Drawing for the job (mm, zero at the part's lowest x, y, z). A direction names the side the tool comes from. Round coordinates to 2 decimals unless told otherwise and drop trailing zeros. Loops run counter-clockwise (first coordinate to the right, second up) from the corner with the lowest first, then second, coordinate; pieces in that order, holes last. Notation, with made-up numbers: M 85.5,30.5 L 113.5,30.5 A8 ccw 113.5,37.5 Z; hole C 21.25,11.25 d3. An arc over 180 degrees is marked long. Use a Markdown table: item, result. Add a question column.
Q1. Cut at A-A (y = 31). Give the cut face in (x, z).
Q2. Tool access for the marked faces 1 and 2: list every direction of +Z, -Z, +X, -X, +Y, -Y with a clear straight run to the whole face (end or side of a thin tool).
Q3. Mould opens along X. For the marked faces 3, 4 and 5 say: +X half, -X half, draft (parallel to the pull), parting line (faces both ways), or undercut.
Q4. Cut at B-B (x = 61.5). Give the cut face in (y, z).
Q5. Probe line 1 (X direction, y = 73.5, z = 45); line 2 (Y direction, x = 60.5, z = 44); line 3 (Z direction, x = 43, y = 35). List the from-to ranges inside material, lowest first. Write a range as from..to.
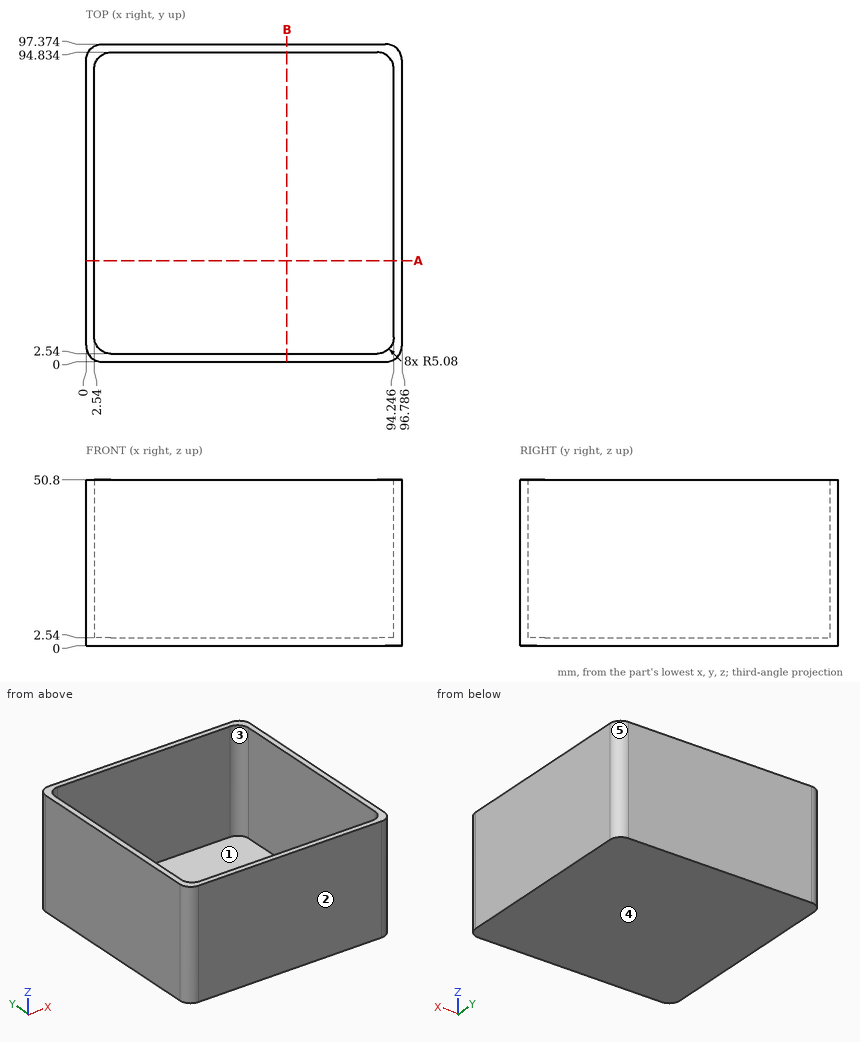
Checked values:
| question | item | result |
|---|---|---|
| 1 | outline | M 0,0 L 96.79,0 L 96.79,50.8 L 94.25,50.8 L 94.25,2.54 L 2.54,2.54 L 2.54,50.8 L 0,50.8 Z |
| 2 | face 1 | +Z |
| 2 | face 2 | +Z, -Z, +X, -X, -Y |
| 3 | face 3 | undercut |
| 3 | face 4 | draft |
| 3 | face 5 | +X half |
| 4 | outline | M 0,0 L 97.37,0 L 97.37,50.8 L 94.83,50.8 L 94.83,2.54 L 2.54,2.54 L 2.54,50.8 L 0,50.8 Z |
| 5 | line 1 | x = 0..2.54, 94.25..96.79 |
| 5 | line 2 | y = 0..2.54, 94.83..97.37 |
| 5 | line 3 | z = 0..2.54 |
